```python
from build123d import *

# Parameters (mm, degrees)
CUT_EXTRUDE1_START = -10
CUT_EXTRUDE1_DEPTH = 10
FILLET3_R          = 0.2
FILLET3_R_2        = 0.5
FILLET3_R_3        = 0.1


with BuildPart() as part:
    # Sketch1 → Revolve1 (revolve)
    with BuildSketch(Plane.XY, mode=Mode.PRIVATE) as revolve1_sk:
        with BuildLine():
            Line((0, 0.8000000000000004), (2, 0.7999999999999999))
            Line((2, 0.7999999999999999), (2, 0.5))
            Line((2, 0.5), (4, 0.5))
            Line((4, 0.5), (4, 0.7999999999999999))
            Line((4, 0.7999999999999999), (18.166969722017665, 0.7999999999999999))
            ThreePointArc((18.166969722017665, 0.7999999999999999), (20.40861928737844, 1.9578126258614066), (22, 0))
            Line((22, 0), (0, 0))
            Line((0, 0), (-2, 0))
            Line((-2, 0), (-2, 0.7999999999999998))
            Line((-2, 0.7999999999999998), (0, 0.8000000000000004))
        make_face()
    revolve(revolve1_sk.sketch.rotate(Axis((0, 0, 0), (1, 0, 0)), 90), axis=Axis((0, 0, 0), (1, 0, 0)))

    # Sketch2 → Cut-Extrude1 (cut)
    with BuildSketch(Plane.ZY.offset(2).offset(CUT_EXTRUDE1_START)):
        with BuildLine():
            Line((0.6244997998398396, -0.5), (-0.6244997998398398, -0.5))
            ThreePointArc((-0.6244997998398398, -0.5), (-1.3e-16, -0.7999999999999998), (0.6244997998398396, -0.5))
        make_face()
        with BuildLine():
            Line((0.6244997998398396, 0.5), (-0.6244997998398398, 0.5))
            ThreePointArc((-0.6244997998398398, 0.5), (-1.3e-16, 0.7999999999999998), (0.6244997998398396, 0.5))
        make_face()
    extrude(amount=CUT_EXTRUDE1_DEPTH, mode=Mode.SUBTRACT)

    # Fillet3
    # the kernel refuses this fillet: 0.5, 0.2, 0.1 mm, written as the material it adds along each edge
    with BuildSketch(Plane(origin=(18.166969722017665, 0, 0), x_dir=(0, 1.1e-16, 1), z_dir=(0, 1, -1.1e-16))) as fillet3_piece_1:
        with BuildLine():
            CenterArc((0.9999999999999997, -0.1265615162442053), FILLET3_R, 117.03569178941255, 62.96430821058948)
            Line((0.7999999999999996, -0.1265615162442124), (0.8, 0))
            ThreePointArc((0.8, 0), (0.8549345824779961, 0.02496864748320604), (0.9090909090909083, 0.05158319232184283))
        make_face()
    revolve(axis=Axis((18.166969722017665, 0, 0), (1, 0, 0)))
    # the kernel refuses this fillet: 0.5, 0.2, 0.1 mm, written as the material it takes off along each edge
    with BuildSketch(Plane(origin=(-2, 0, 0), x_dir=(0, 0.7854961071297899, -0.6188665976476235), z_dir=(0, -0.6188665976476235, -0.7854961071297899))) as fillet3_2_piece_1:
        with BuildLine():
            CenterArc((0.7999999999999998 - FILLET3_R_2, FILLET3_R_2), FILLET3_R_2, 270, 90)
            Line((0.7999999999999998 - FILLET3_R_2, 0), (0.7999999999999998, 0))
            Line((0.7999999999999998, 0), (0.7999999999999998, FILLET3_R_2))
        make_face()
    revolve(axis=Axis((-2, 0, 0), (1, 0, 0)), revolution_arc=256.4668291762195, mode=Mode.SUBTRACT)
    with BuildSketch(Plane(origin=(-2, 0, 0), x_dir=(0, -0.7854961071297903, 0.6188665976476231), z_dir=(0, 0.6188665976476231, 0.7854961071297903))) as fillet3_2_piece_2:
        with BuildLine():
            CenterArc((0.7999999999999998 - FILLET3_R_2, FILLET3_R_2), FILLET3_R_2, 270, 90)
            Line((0.7999999999999998 - FILLET3_R_2, 0), (0.7999999999999998, 0))
            Line((0.7999999999999998, 0), (0.7999999999999998, FILLET3_R_2))
        make_face()
    revolve(axis=Axis((-2, 0, 0), (1, 0, 0)), revolution_arc=256.46682917621945, mode=Mode.SUBTRACT)
    with BuildSketch(Plane(origin=(8, 6.7e-16, -1.1e-16), x_dir=(0, -0.35458319650881664, -0.9350244685320219), z_dir=(0, 0.9350244685320219, -0.35458319650881664))) as fillet3_2_piece_3_section:
        with BuildLine():
            CenterArc((0.8000000000000002 - FILLET3_R_3, -FILLET3_R_3), FILLET3_R_3, 0, 90)
            Line((0.8000000000000002 - FILLET3_R_3, 0), (0.8000000000000002, 0))
            Line((0.8000000000000002, 0), (0.8000000000000002, -FILLET3_R_3))
        make_face()
    fillet3_2_piece_3 = revolve(axis=Axis((8, 6.7e-16, -1.1e-16), (-1, 0, 0)), revolution_arc=138.4641967481308, mode=Mode.PRIVATE)
    fillet3_2_piece_3 = split(fillet3_2_piece_3, bisect_by=Plane(origin=(8.02822018538669, -0.5, -2.2e-16), z_dir=(0, -1, 0)), keep=Keep.TOP, mode=Mode.PRIVATE)
    add(fillet3_2_piece_3, mode=Mode.SUBTRACT)
    with BuildSketch(Plane(origin=(8, -6.7e-16, -1.1e-16), x_dir=(0, 0.35458319650881664, -0.9350244685320219), z_dir=(0, -0.9350244685320219, -0.35458319650881664))) as fillet3_2_piece_4_section:
        with BuildLine():
            CenterArc((0.8 - FILLET3_R_3, FILLET3_R_3), FILLET3_R_3, 270, 90)
            Line((0.8 - FILLET3_R_3, 0), (0.8, 0))
            Line((0.8, 0), (0.8, FILLET3_R_3))
        make_face()
    fillet3_2_piece_4 = revolve(axis=Axis((8, -6.7e-16, -1.1e-16), (1, 0, 0)), revolution_arc=138.4641967481308, mode=Mode.PRIVATE)
    fillet3_2_piece_4 = split(fillet3_2_piece_4, bisect_by=Plane(origin=(8.02822018538669, 0.5, -2.2e-16), z_dir=(0, 1, 0)), keep=Keep.TOP, mode=Mode.PRIVATE)
    add(fillet3_2_piece_4, mode=Mode.SUBTRACT)


solid = part.part
```
Could you check a few things on this model? Use its own coordinates, in mm. A direction names the side the tool comes from. Round coordinates to 2 decimals unless told otherwise and drop trailing zeros. Write each loop counter-clockwise with the first axis right and the second up, starting at its lowest first coordinate (ties: lowest second). Pieces come first, ordered by that corner, then holes. Notation, with made-up numbers: M 6,-34 L 48,-34 A34 cw 48,-4 Z; hole C -2,36 d9. An arc over 180 degrees is marked long. Answer in a Markdown table with one row per item. Add a question column.
Q1. Imagine slicing it at A-A (z = 1.2). Please give me the cut outline in (x, y).
Q2. If I drill on line 1 (Y direction, x = 13.25, z = 0); line 2 (Z direction, x = 18, y = -0.5); line 3 (X direction, y = -0.45, z = 0.5), over which ranges is the centre line in solid material (lowest first)? Write a range as from..to.
Q3. If we mould it in two halves opening along X, with no side actions, what happens to faces 4 (the cylindrical face through (3.014, 0.488, -0.108)), 5 (the cylindrical face through (0.3, 0, -0.8))? For each: +X half, -X half, draft (parallel to the pull), parting line (faces both ways), or undercut.
Q4. Will these pins go through, and if not, where does the flat tip stop? pin 1 Ø1.4 at (x, z) = (0, 0) entering from +Y; pin 2 Ø0.6 at (y, z) = (0, 0.5) entering from +X; pin 3 Ø2 at (x, y) = (14, -0.5) entering from -Z.
Q5. Imagine slicing it at B-B (x = 16). Please give me the cut outline in (y, z).
Q6. On a 3-axis mill with a long thin cutter (end or side, diameter ignored), from which of +Z, -Z, +X, -X, +Y, -Y can I reach the whole of each face in a straight line? I mean faces 1 (the cylindrical face through (12.68, 0.71, 0.37)), 2 (the cylindrical face through (0.3, 0, 0.8)), 3 (the flat face through (0, -0.5, 0)). Say none if no direction works.
Values:
| question | item | result |
|---|---|---|
| 1 | outline | C 20,0 d3.2 |
| 2 | line 1 | -0.8..0.8 |
| 2 | line 2 | -0.62..0.62 |
| 2 | line 3 | -1.83..2, 4..21.88 |
| 3 | face 4 | undercut |
| 3 | face 5 | draft |
| 4 | pin 1 | y = 0.5 |
| 4 | pin 2 | x = 21.99 |
| 4 | pin 3 | z = -0.8 |
| 5 | outline | C 0,0 d1.6 |
| 6 | face 1 | -X |
| 6 | face 2 | +Z, -X |
| 6 | face 3 | +Z, -Z, -X, -Y |
